from build123d import *

# Parameters (mm, degrees)
SKETCH1_W           = 48
SKETCH1_H           = 22
SKETCH1_R           = 5
SKETCH1_R_2         = 1
BOSS_EXTRUDE1_DEPTH = 3
SKETCH1_2_R         = 5
BOSS_EXTRUDE2_DEPTH = 8
SKETCH2_W           = 2.104353458
SKETCH2_H           = 1.008785287
SKETCH2_W_2         = 1.832797116
SKETCH2_W_3         = 2.088179476
SKETCH2_W_4         = 0.74441479
SKETCH2_H_2         = 2.033036387
SKETCH2_W_5         = 0.836105694
SKETCH2_W_6         = 1.094706322
BOSS_EXTRUDE3_DEPTH = 0.5
SKETCH2_3_W         = 4.22759305
SKETCH2_3_H         = 1.274477447
SKETCH2_3_W_2       = 3.360802222
SKETCH2_3_H_2       = 1.472211858
SKETCH2_3_W_3       = 1.045429968
SKETCH2_3_H_3       = 1.557369002
SKETCH2_3_W_4       = 1.219219908
SKETCH2_3_H_4       = 2.19777591
SKETCH2_3_W_5       = 1.132324938
SKETCH2_3_H_5       = 1.302990818
BOSS_EXTRUDE4_DEPTH = 0.8
SKETCH2_4_W         = 10.139826511
SKETCH2_4_H         = 3.693874046
BOSS_EXTRUDE5_DEPTH = 1.2
SKETCH2_5_R         = 1.302990818
SKETCH2_5_R_2       = 1.47373415
BOSS_EXTRUDE6_DEPTH = 1.5
SKETCH4_R           = 5.057320887
BOSS_EXTRUDE7_DEPTH = 1


with BuildPart() as part:
    # Sketch1 → Boss-Extrude1 (new body)
    with BuildSketch(Plane(origin=(0, 0, 0), x_dir=(0, 0, -1), z_dir=(1, 0, 0))):
        with Locations((24, 11)):
            Rectangle(SKETCH1_W, SKETCH1_H)
        with Locations((38, 9.99550505)):
            Circle(SKETCH1_R, mode=Mode.SUBTRACT)
        with Locations((40.65, 18.99550505)):
            Circle(SKETCH1_R_2, mode=Mode.SUBTRACT)
        with Locations((2.4, 18.99550505)):
            Circle(SKETCH1_R_2, mode=Mode.SUBTRACT)
        with Locations((2, 1.2)):
            Circle(SKETCH1_R_2, mode=Mode.SUBTRACT)
        with Locations((40.25, 1.2)):
            Circle(SKETCH1_R_2, mode=Mode.SUBTRACT)
    extrude(amount=BOSS_EXTRUDE1_DEPTH)

    # Sketch1_2 → Boss-Extrude2 (add)
    with BuildSketch(Plane(origin=(0, 0, 0), x_dir=(0, 0, -1), z_dir=(1, 0, 0))):
        with Locations((38, 9.99550505)):
            Circle(SKETCH1_2_R)
    extrude(amount=BOSS_EXTRUDE2_DEPTH)

    # Sketch2 → Boss-Extrude3 (add)
    with BuildSketch(Plane.ZY):
        with Locations((-16.200734104, 17.368839016)):
            Rectangle(SKETCH2_W, SKETCH2_H)
        with Locations((-12.333531989, 17.368839016)):
            Rectangle(SKETCH2_W_2, SKETCH2_H)
        with Locations((-7.896046505, 17.368839016)):
            Rectangle(SKETCH2_W_3, SKETCH2_H)
        with Locations((-27.104604618, 3.695463372)):
            Rectangle(SKETCH2_W_4, SKETCH2_H_2)
        with Locations((-29.462717027, 3.695463372)):
            Rectangle(SKETCH2_W_5, SKETCH2_H_2)
        with Locations((-32.481789363, 3.695463372)):
            Rectangle(SKETCH2_W_6, SKETCH2_H_2)
    extrude(amount=BOSS_EXTRUDE3_DEPTH)

    # Sketch2_3 → Boss-Extrude4 (add)
    with BuildSketch(Plane.ZY):
        with Locations((-13.530929956, 8.546365696)):
            Rectangle(SKETCH2_3_W, SKETCH2_3_H)
        with Locations((-4.603155303, 7.810259766)):
            Rectangle(SKETCH2_3_W_2, SKETCH2_3_H_2)
        with Locations((-46.592324849, 9.96228892)):
            Rectangle(SKETCH2_3_W_3, SKETCH2_3_H_3)
        with Locations((-45.982714895, 4.794351326)):
            Rectangle(SKETCH2_3_W_4, SKETCH2_3_H_4)
        with Locations((-46.548877364, 2.027449769)):
            Rectangle(SKETCH2_3_W_5, SKETCH2_3_H_5)
    extrude(amount=BOSS_EXTRUDE4_DEPTH)

    # Sketch2_4 → Boss-Extrude5 (add)
    with BuildSketch(Plane.ZY):
        with Locations((-26.864522947, 12.587910444)):
            Rectangle(SKETCH2_4_W, SKETCH2_4_H)
    extrude(amount=BOSS_EXTRUDE5_DEPTH)

    # Sketch2_5 → Boss-Extrude6 (add)
    with BuildSketch(Plane.ZY):
        with Locations((-6.851956767, 2.678945178)):
            Circle(SKETCH2_5_R)
        with Locations((-15.644726481, 4.711981565)):
            Circle(SKETCH2_5_R_2)
    extrude(amount=BOSS_EXTRUDE6_DEPTH)

    # Sketch4 → Boss-Extrude7 (add)
    with BuildSketch(Plane(origin=(8, 0, 0), x_dir=(0, 0, -1), z_dir=(1, 0, 0))):
        with Locations((37.964303181, 10.142557879)):
            Circle(SKETCH4_R)
    extrude(amount=BOSS_EXTRUDE7_DEPTH)


solid = part.part
CAD build for the part. Positions are in the model's coordinates, mm. A direction names the side the tool comes from. Round coordinates to 2 decimals unless told otherwise and drop trailing zeros. Write each loop counter-clockwise with the first axis right and the second up, starting at its lowest first coordinate (ties: lowest second). Pieces come first, ordered by that corner, then holes. Notation, with made-up numbers: (75.5, 42.25) -> (84.5, 42.25) arc R36 ccw to (84.5, 77.25) -> close; hole circle Ø2 at (83, 33). An arc over 180 degrees is marked (long way). Answer as a JSON object with one key per item and string values.
(1) Band-saw the part on D-D, the plane x = 5.5. List the corners of the cut face in (y, z).
Reported:
{"outline": "circle Ø10 at (10, -38)"}
(2) Pin check, flat tips, straight feed: P1, Ø6, axis at x = 7.5, z = -20.5, coming from the -Y side; P2, Ø0.8, axis at y = 17, z = -16.5, coming from the -X side; P3, Ø0.9, axis at x = -0.5, y = 7.5, coming from the -Z side; P4, Ø0.6, axis at x = -0.5, y = 12.5, coming from the +Z side. Stop position of each tip, or through.
Reported:
{"P1": "passes through", "P2": "stops at x = -0.5", "P3": "stops at z = -15.64", "P4": "stops at z = -21.79"}
(3) Band-saw the part on A-A, the plane z = -40.65. List the corners of the cut face in (x, y).
Reported:
{"outline": "(0, 0) -> (3, 0) -> (3, 0.28) -> (0, 0.28) -> close; (0, 2.12) -> (3, 2.12) -> (3, 5.76) -> (8, 5.76) -> (8, 5.86) -> (9, 5.86) -> (9, 14.43) -> (8, 14.43) -> (8, 14.24) -> (3, 14.24) -> (3, 18) -> (0, 18) -> close; (0, 20) -> (3, 20) -> (3, 22) -> (0, 22) -> close"}
(4) Band-saw the part on C-C, the plane z = -2. List the corners of the cut face in (x, y), then the cut area to 3 significant figures.
Reported:
{"outline": "(0, 0) -> (3, 0) -> (3, 0.2) -> (0, 0.2) -> close; (0, 2.2) -> (3, 2.2) -> (3, 18.08) -> (0, 18.08) -> close; (0, 19.91) -> (3, 19.91) -> (3, 22) -> (0, 22) -> close", "area": "54.5 mm^2"}
(5) Band-saw the part on B-B, the plane z = -10.5. List the corners of the cut face in (x, y), then the cut area to 3 significant figures.
Reported:
{"outline": "(0, 0) -> (3, 0) -> (3, 22) -> (0, 22) -> close", "area": "66.0 mm^2"}
(6) Probe probe 1 along Y at (x, z) = (1.4, -40.25); probe 2 along Y at (x, z) = (1.35, -40.65); probe 3 along X at (y, z) = (15, -37). List the from-to ranges inside material, lowest first. Write a range as [from, to].
Reported:
{"probe 1": "y = [0, 0.2], [2.2, 18.08], [19.91, 22]", "probe 2": "y = [0, 0.28], [2.12, 18], [20, 22]", "probe 3": "x = [0, 3], [8, 9]"}
(7) Which spindle directions (+Z, -Z, +X, -X, +Y, -Y) get a long thin tool onto all of the face, cutting with end or side? Do faces 1 (the face through (-0.74, 3.778, -6.151)), 2 (the face through (-0.8, 5, -46)), 3 (the face through (-0.5, 17.4, -7.9)). Say none if no direction does.
Reported:
{"face 1": "-X", "face 2": "-Z, -X, +Y, -Y", "face 3": "+Z, -Z, -X, +Y"}
(8) Two-plate mould, pull along X, no slides. Class faces 4 (the face through (9, 10, -38)), 5 (the face through (5, 10, -33)), 6 (the face through (-0.5, 17.4, -12.3)): +X half, -X half, draft (parallel to the pull), parting line (faces both ways), or undercut.
Reported:
{"face 4": "+X half", "face 5": "undercut", "face 6": "-X half"}
